Print and shaded views of the part. All mm, measured from the part's lowest x, y and z. Give positions to 0.01 mm unless a question says otherwise; leave off trailing zeros. Loops run counter-clockwise (first coordinate to the right, second up) from the corner with the lowest first, then second, coordinate; pieces in that order, holes last. Notation, with made-up numbers: (71, -14) - (104, -14) arc R7 ccw to (104, -1) - close; hole circle Ø4 at (24, 23.5). An arc over 180 degrees is marked (long way). Return JSON: item names as keys, results as strings.
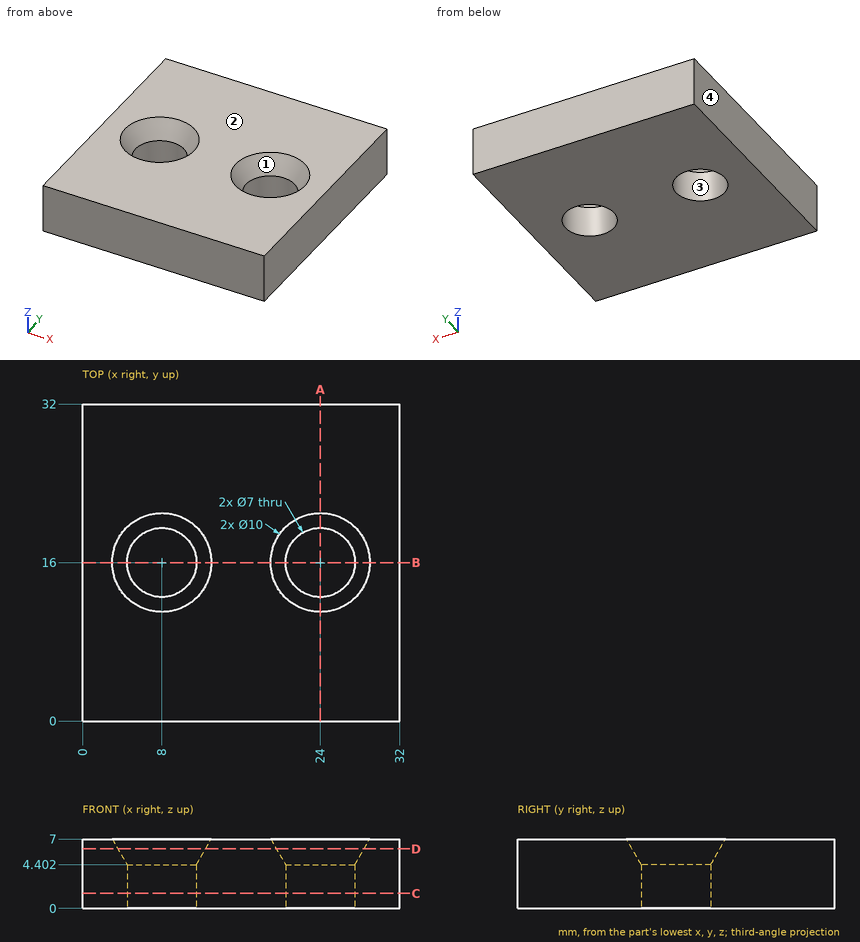
1. Cut at B-B, the plane y = 16. Write the cut outline in (x, z), plus the area to 3 significant figures.
Values follow:
{"outline": "(0, 0) - (4.5, 0) - (4.5, 4.4) - (3, 7) - (0, 7) - close; (11.5, 0) - (20.5, 0) - (20.5, 4.4) - (19, 7) - (13, 7) - (11.5, 4.4) - close; (27.5, 0) - (32, 0) - (32, 7) - (29, 7) - (27.5, 4.4) - close", "area": "118 mm²"}
2. Drill centre lines: probe 1 along X at (y, z) = (16, 0.95); probe 2 along Y at (x, z) = (24, 1.2); probe 3 along Y at (x, z) = (22.5, 3.5). Where is each one in solid material? Low to high.
Values follow:
{"probe 1": "x = 0 to 4.5, 11.5 to 20.5, 27.5 to 32", "probe 2": "y = 0 to 12.5, 19.5 to 32", "probe 3": "y = 0 to 12.84, 19.16 to 32"}
3. Pull direction X, two halves, no side cores. Call the marked faces 1, 2, 3 and 4: +X half, -X half, draft (parallel to the pull), parting line (faces both ways), or undercut.
Values follow:
{"face 1": "undercut", "face 2": "draft", "face 3": "undercut", "face 4": "-X half"}
4. Cut at D-D, the plane z = 6. Write the cut outline in (x, y), plus the area to 3 significant figures.
Values follow:
{"outline": "(0, 0) - (32, 0) - (32, 32) - (0, 32) - close; hole circle Ø8.85 at (8, 16); hole circle Ø8.85 at (24, 16)", "area": "901 mm²"}
5. Drop a flat-ended pin along its axis: P1, Ø5, axis at x = 10, y = 9.5, coming from the -Z side. Give the stop position or say it passes through.
Values follow:
{"P1": "stops at z = 0"}
6. Cut at A-A, the plane x = 24. Write the cut outline in (y, z), plus the area to 3 significant figures.
Values follow:
{"outline": "(0, 0) - (12.5, 0) - (12.5, 4.4) - (11, 7) - (0, 7) - close; (19.5, 0) - (32, 0) - (32, 7) - (21, 7) - (19.5, 4.4) - close", "area": "171 mm²"}
7. Cut at C-C, the plane z = 1.5. Write the cut outline in (x, y), plus the area to 3 significant figures.
Values follow:
{"outline": "(0, 0) - (32, 0) - (32, 32) - (0, 32) - close; hole circle Ø7 at (8, 16); hole circle Ø7 at (24, 16)", "area": "947 mm²"}
